```python
from build123d import *

# Parameters (mm, degrees)
F1_DEPTH       = 20
F3_DEPTH       = 15
F5_D           = 6.3
F5_DEPTH       = 30
F5_TIP         = 1.8927109499
F6_DEPTH       = 5
F8_D           = 6.6
F8_DEPTH       = 21
F8_START       = 18.1600674
F8_CBORE_D     = 12.5
F8_CBORE_DEPTH = 12
F8_TIP         = 1.9828400428
F9_T1_DEPTH    = 66.2237980807
F9_T3_DEPTH    = 48.9219521717
F10_SIZE       = 10


# Not quite as in the source:
# - a fillet or chamfer that OpenCascade refuses, or shapes differently, is made with other operations: its cross-section is extruded or revolved along the edge and cut away or added


with BuildPart() as f1:
    # F0 (on Right) → F1 (new body)
    with BuildSketch(Plane.YZ):
        Polygon((-16.375976861, 0), (-16.375976861, 10), (-16.375976861, 15), (16.375976861, 15), (16.375976861, 10), (16.375976861, 0), (40, 0), (40, 15.2900453504), (12.5, 35), (0, 35), (-12.5, 35), (-40, 15.2900453504), (-40, 0), align=None)
    extrude(amount=-F1_DEPTH)

    # F2 (on face) → F3 (join)
    with BuildSketch(Plane.YZ):
        with BuildLine():
            ThreePointArc((0, 17.0022554452), (5.6591519034, 19.3441438406), (8.0035544985, 25.0022546555))
            ThreePointArc((8.0035544985, 25.0022546555), (5.6591519034, 30.6603654705), (0, 33.0022538659))
            Line((0, 33.0022538659), (0, 17.0022554452))
        make_face()
        with BuildLine():
            Line((0, 17.0022554452), (0, 33.0022538659))
            ThreePointArc((0, 33.0022538659), (-7.9964455015, 25.0022546555), (0, 17.0022554452))
        make_face()
    extrude(amount=F3_DEPTH)

    # F5
    with Locations(Plane.YZ.offset(15)):
        with Locations((0.0035544985, 25.0022546555)):
            Hole(F5_D / 2, depth=F5_DEPTH)
            with Locations((0, 0, -(F5_DEPTH + F5_TIP / 2))):  # 118° drill point
                Cone(0, F5_D / 2, F5_TIP, mode=Mode.SUBTRACT)

    # F4 (on face) → F6 (cut)
    with BuildSketch(Plane.YZ.offset(15)):
        Polygon((5.1826206219, 28.040446128), (-0.0380634364, 31.0065532225), (-5.2171295598, 27.9683617501), (-5.1755116248, 21.9640631831), (0.0451724335, 18.9979560886), (5.2242385569, 22.036147561), align=None)
    extrude(amount=-F6_DEPTH, mode=Mode.SUBTRACT)

    # F8
    # its depths count from where the whole tool has entered the part; down to there all is cleared
    with Locations(Plane.XY.offset(35).offset(-F8_START)):
        with Locations((-10, 31.5875445392), (-10, -31.5875445392)):
            CounterBoreHole(F8_D / 2, F8_CBORE_D / 2, F8_CBORE_DEPTH, depth=F8_DEPTH)
            with Locations((0, 0, -(F8_DEPTH + F8_TIP / 2))):  # 118° drill point
                Cone(0, F8_D / 2, F8_TIP, mode=Mode.SUBTRACT)

    # F9: fillet of radius 18 on 4 edges, made by hand

    # F9_s2 → F9_t1 (cut)
    with BuildSketch(Plane.YZ.offset(-43.1118990403)):
        with BuildLine():
            ThreePointArc((40, 6.0452857343), (38.0116581667, 14.2688374458), (32.4859108054, 20.6755856144))
            Line((32.4859108054, 20.6755856144), (40, 15.2900453504))
            Line((40, 15.2900453504), (40, 6.0452857343))
        make_face()
        with BuildLine():
            ThreePointArc((-40, 6.0452857343), (-38.0116581667, 14.2688374458), (-32.4859108054, 20.6755856144))
            Line((-32.4859108054, 20.6755856144), (-40, 15.2900453504))
            Line((-40, 15.2900453504), (-40, 6.0452857343))
        make_face()
    extrude(amount=F9_T1_DEPTH, mode=Mode.SUBTRACT)

    # F9_s4 → F9_t3 (cut)
    with BuildSketch(Plane.YZ.offset(-34.4609760859)):
        with BuildLine():
            ThreePointArc((17.201520371, 31.6302998801), (12.2226324527, 34.1368812484), (6.7156095657, 35))
            Line((6.7156095657, 35), (12.5, 35))
            Line((12.5, 35), (17.201520371, 31.6302998801))
        make_face()
        with BuildLine():
            ThreePointArc((-6.7156095657, 35), (-12.2226324527, 34.1368812484), (-17.201520371, 31.6302998801))
            Line((-17.201520371, 31.6302998801), (-12.5, 35))
            Line((-12.5, 35), (-6.7156095657, 35))
        make_face()
    extrude(amount=F9_T3_DEPTH, mode=Mode.SUBTRACT)

    # F10
    f10_edges = [f1.edges().sort_by_distance(p)[0] for p in [
        (-10, 16.375977, 15),
        (-10, -16.375977, 15),
    ]]
    chamfer(f10_edges, length=F10_SIZE)


solid = f1.part
```
For this review, take the finished solid that the model builds, in its own axes (mm). A direction names the side the tool comes from. Round coordinates to 2 decimals unless told otherwise and drop trailing zeros. Write each loop counter-clockwise with the first axis right and the second up, starting at its lowest first coordinate (ties: lowest second). Pieces come first, ordered by that corner, then holes. Notation, with made-up numbers: (87.25, 79) -> (146.25, 79) arc R19 cw to (146.25, 94) -> close; hole circle Ø5 at (3, 64.25). An arc over 180 degrees is marked (long way). One line per question, with ' | ' between items. Start each with the question number.
(1) Add section A-A, the plane z = 10.5. Write out the cut boundary in (x, y), plus the area to 3 significant figures.
(2) Add section D-D, the plane y = -12. Write out the cut boundary in (x, z).
(3) Mouldability with a two-part tool opening along Z and no side actions: class faces 1 (the face through (-10, 40, 3)), 2 (the face through (10, -2, 22)), 3 (the face through (-9.86, 11.446, 9.93)), 4 (the face through (12.535, 2.598, 20.496)) as released by +Z, released by -Z, zero draft, split by the parting line, or undercut.
(4) Add section C-C, the plane x = -5. Write out the cut boundary in (y, z), plus the area to 3 significant figures.
(5) Insertion check: P1, Ø12, axis at x = 7, z = 27.5, coming from the +Y side; P2, Ø10, axis at x = -12, z = 15.5, coming from the +Y side; P3, Ø14, axis at x = -6, y = 1, coming from the -Z side. Each pin has a flat end and moves straight along its axis. Give the tip position at first contact, or say it passes through.
(6) Add section B-B, the plane x = -10.5. Give the number of separate pieces and of enclosed holes in the cut face, plus the area to 3 significant figures.
(7) For line 1 along Y through (x, z) = (-5, 14.5); line 2 along Y through (x, z) = (-16, 4.5); line 3 along Y through (x, z) = (-10, 12), list the stretches that pass through material, from the lowest coordinate up. Write a range as from..to.
(8) Tool access review of faces 5 (the face through (-9.86, -11.306, 10.07)), 6 (the face through (12.54, -2.59, 29.51)), 7 (the face through (-10.81, -25.39, 13.14)): name each direction out of +Z, -Z, +X, -X, +Y, -Y from which nothing blocks a thin tool from reaching the whole face with its end or side.
Answer list:
1) outline: (-20, -39.44) -> (0, -39.44) -> (0, -10.88) -> (-20, -10.88) -> close; (-20, 10.88) -> (0, 10.88) -> (0, 39.44) -> (-20, 39.44) -> close; hole circle Ø12.5 at (-10, -31.59); hole circle Ø12.5 at (-10, 31.59) | area: 897 mm²
2) outline: (-20, 9.38) -> (0, 9.38) -> (0, 34.21) -> (-20, 34.21) -> close
3) face 1: zero draft | face 2: undercut | face 3: released by -Z | face 4: undercut
4) outline: (-40, 0) -> (-16.38, 0) -> (-16.38, 5) -> (-6.38, 15) -> (6.38, 15) -> (16.38, 5) -> (16.38, 0) -> (40, 0) -> (40, 6.05) arc R18 ccw to (35.34, 18.13) -> (35.34, 4.84) -> (27.84, 4.84) -> (27.84, 24.01) -> (17.2, 31.63) arc R18 ccw to (6.72, 35) -> (-6.72, 35) arc R18 ccw to (-17.2, 31.63) -> (-27.84, 24.01) -> (-27.84, 4.84) -> (-35.34, 4.84) -> (-35.34, 18.13) arc R18 ccw to (-40, 6.05) -> close; hole circle Ø6.3 at (0, 25) | area: 1,560 mm²
5) P1: y = 8 | P2: y = 39.44 | P3: z = 13.38
6) separate pieces: 3 | enclosed holes: 1 | area: 1,340 mm²
7) line 1: -37.89..-35.34, -27.84..-6.88, 6.88..27.84, 35.34..37.89 | line 2: -40..-16.38, 16.38..40 | line 3: -38.99..-37.84, -25.34..-9.38, 9.38..25.34, 37.84..38.99
8) face 5: -Z, +X, -X | face 6: +X | face 7: +Z
